Source: three-view drawing plus pictorial views. Frame: mm from the lowest corner of the part. A direction names the side the tool comes from. Round coordinates to 2 decimals unless told otherwise and drop trailing zeros. Loops run counter-clockwise (first coordinate to the right, second up) from the corner with the lowest first, then second, coordinate; pieces in that order, holes last. Notation, with made-up numbers: (12, 73.5) -> (30, 73.5) arc R29 ccw to (30, 101.5) -> close; hole circle Ø7 at (56.25, -9.75). An arc over 180 degrees is marked (long way). Answer in a Markdown table with one row per item. Add a question column.
Q1. Section D-D, the plane y = 11. Output: boundary loops of the cut face in (x, z).
Q2. Section C-C, the plane z = 7.5. Output: boundary loops of the cut face in (x, y), and give its area (3 significant figures).
Q3. Section A-A, the plane y = 14. Output: boundary loops of the cut face in (x, z), and give its area (3 significant figures).
Q4. Pin query (flat end, axial travel): pin 1 (3 mm diameter, centred on y = 5.5, z = 2.5, fed in from -X); pin 2 (2 mm diameter, centred on y = 9.5, z = 5.5, fed in from +X); pin 3 (3 mm diameter, centred on y = 22, z = 2, fed in from -X); pin 4 (4 mm diameter, centred on x = 14, y = 17, fed in from -Z). Return the tip coordinate at first contact, or that it passes through.
Q5. Mould query, pull axis X, two halves, no side actions, for the marked faces 4, 5 and 6. Classes: pulls with the +X half, pulls with the -X half, needs draft (parallel to the pull), parting line crosses it, or undercut.
Q6. Reachability of the marked faces 1, 2 and 3 from +Z, -Z, +X, -X, +Y, -Y: full face, straight path, thin tool, end or side. Return the list, or none.
Q7. Section B-B, the plane x = 14. Output: boundary loops of the cut face in (y, z), and give its area (3 significant figures).
Q8. Ray query, L1, parallel to Y at x = 14, z = 2.75; L2, parallel to Y at x = 14, z = 4.75; L3, parallel to Z at x = 16.25, y = 3.25. Return the intervals inside material, ascending. Write a range as from..to.
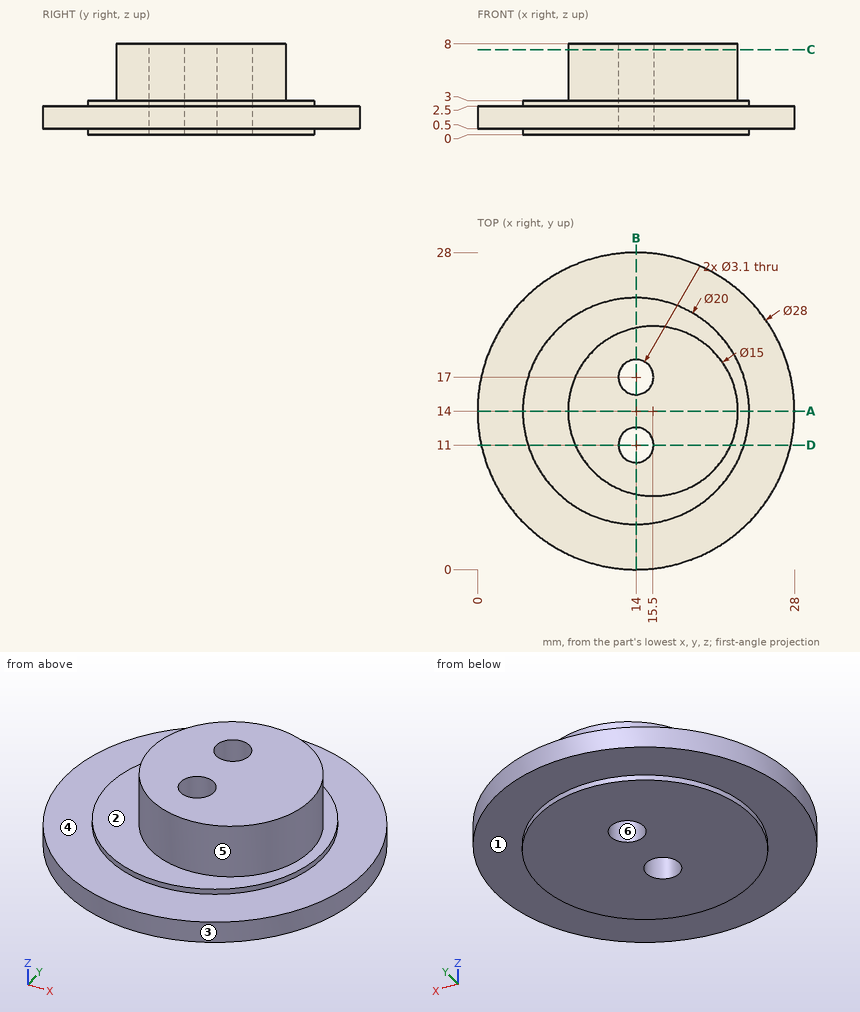
Answer block:
| question | item | result |
|---|---|---|
| 1 | outline | (0.33, 0.5) -> (4.46, 0.5) -> (4.46, 0) -> (12.45, 0) -> (12.45, 8) -> (8.63, 8) -> (8.63, 3) -> (4.46, 3) -> (4.46, 2.5) -> (0.33, 2.5) -> close; (15.55, 0) -> (23.54, 0) -> (23.54, 0.5) -> (27.67, 0.5) -> (27.67, 2.5) -> (23.54, 2.5) -> (23.54, 3) -> (22.37, 3) -> (22.37, 8) -> (15.55, 8) -> close |
| 2 | outline | circle Ø15 at (15.5, 14); hole circle Ø3.1 at (14, 11); hole circle Ø3.1 at (14, 17) |
| 2 | area | 162 mm^2 |
| 3 | outline | (0, 0.5) -> (4, 0.5) -> (4, 0) -> (24, 0) -> (24, 0.5) -> (28, 0.5) -> (28, 2.5) -> (24, 2.5) -> (24, 3) -> (23, 3) -> (23, 8) -> (8, 8) -> (8, 3) -> (4, 3) -> (4, 2.5) -> (0, 2.5) -> close |
| 3 | area | 151 mm^2 |
| 4 | pin 1 | x = 1.88 |
| 4 | pin 2 | x = 22.13 |
| 4 | pin 3 | x = 1.6 |
| 4 | pin 4 | z = 0 |
| 5 | face 4 | needs draft |
| 5 | face 5 | parting line crosses it |
| 5 | face 6 | undercut |
| 6 | face 1 | -Z |
| 6 | face 2 | +Z |
| 6 | face 3 | +Z, -Z |
| 7 | outline | (0, 0.5) -> (4, 0.5) -> (4, 0) -> (9.45, 0) -> (9.45, 8) -> (6.65, 8) -> (6.65, 3) -> (4, 3) -> (4, 2.5) -> (0, 2.5) -> close; (12.55, 0) -> (15.45, 0) -> (15.45, 8) -> (12.55, 8) -> close; (18.55, 0) -> (24, 0) -> (24, 0.5) -> (28, 0.5) -> (28, 2.5) -> (24, 2.5) -> (24, 3) -> (21.35, 3) -> (21.35, 8) -> (18.55, 8) -> close |
| 7 | area | 99.9 mm^2 |
| 8 | L1 | 4..9.45, 12.55..15.45, 18.55..24 |
| 8 | L2 | 6.65..9.45, 12.55..15.45, 18.55..21.35 |
| 8 | L3 | 0.5..2.5 |
